Design review of the part built by this model. Coordinates are the model's own, in mm. A direction names the side the tool comes from. Coordinates: 2 decimals unless noted, no trailing zeros. Write each loop counter-clockwise with the first axis right and the second up, starting at its lowest first coordinate (ties: lowest second). Pieces come first, ordered by that corner, then holes. Notation, with made-up numbers: M -22.75,33 L 12.25,33 A26 cw 12.25,48 Z; hole C 35.25,-4 d7. An arc over 180 degrees is marked long. One line per question, with ' | ' between items.
from build123d import *

# Parameters (mm, degrees)
SKETCH1_W            = 30
SKETCH1_H            = 5
BOSS_EXTRUDE1_DEPTH  = 19.3
SKETCH2_W            = 40
SKETCH2_H            = 10
BOSS_EXTRUDE2_DEPTH  = 3.175
SKETCH3_W            = 4
SKETCH3_H            = 30
BOSS_EXTRUDE3_DEPTH  = 75
CUT_EXTRUDE1_REACH   = 84.48
SKETCH4_R            = 7.1
BOSS_EXTRUDE7_DEPTH  = 5
BOSS_EXTRUDE8_DEPTH  = 5
CHAMFER1_SIZE        = 5
BOSS_EXTRUDE9_DEPTH  = 75
BOSS_EXTRUDE10_DEPTH = 5
CHAMFER2_SIZE        = 5
CHAMFER3_SIZE        = 10
BOSS_EXTRUDE15_DEPTH = 3.175
CUT_EXTRUDE2_DEPTH   = 81.759021382
FILLET6_R            = 1
FILLET7_R            = 1
CHAMFER6_SIZE        = 2.5


with BuildPart() as part:
    # Sketch1 → Boss-Extrude1 (new body)
    with BuildSketch(Plane(origin=(0, 0, 0), x_dir=(0, 0, -1), z_dir=(1, 0, 0))):
        Rectangle(SKETCH1_W, SKETCH1_H)
    extrude(amount=BOSS_EXTRUDE1_DEPTH)

    # Sketch2 → Boss-Extrude2 (add)
    with BuildSketch(Plane.ZY):
        with Locations((0.597390222, 2.5)):
            Rectangle(SKETCH2_W, SKETCH2_H)
    extrude(amount=-BOSS_EXTRUDE2_DEPTH)

    # Sketch3 → Boss-Extrude3 (add)
    with BuildSketch(Plane.XZ.offset(2.5)):
        with Locations((17.3, 0)):
            Rectangle(SKETCH3_W, SKETCH3_H)
    extrude(amount=BOSS_EXTRUDE3_DEPTH)

    # Sketch4 → Cut-Extrude1 (cut, up to next)
    with BuildSketch(Plane(origin=(19.3, 0, 0), x_dir=(0, 0, -1), z_dir=(1, 0, 0)), mode=Mode.PRIVATE) as cut_extrude1_sk1:
        with Locations((2.035e-06, -17.9)):
            Circle(SKETCH4_R)
    cut_extrude1_tool1 = extrude(cut_extrude1_sk1.sketch, amount=-CUT_EXTRUDE1_REACH, mode=Mode.PRIVATE) & part.part
    # Sketch4 → Cut-Extrude1 (cut, up to next)
    with BuildSketch(Plane(origin=(19.3, 0, 0), x_dir=(0, 0, -1), z_dir=(1, 0, 0)), mode=Mode.PRIVATE) as cut_extrude1_sk2:
        with Locations((-1.3e-07, -65.9)):
            Circle(SKETCH4_R)
    cut_extrude1_tool2 = extrude(cut_extrude1_sk2.sketch, amount=-CUT_EXTRUDE1_REACH, mode=Mode.PRIVATE) & part.part
    add(cut_extrude1_tool1.solids().sort_by_distance((19.3, -17.9, -2e-06))[0], mode=Mode.SUBTRACT)
    add(cut_extrude1_tool2.solids().sort_by_distance((19.3, -65.9, 0))[0], mode=Mode.SUBTRACT)

    # Sketch10 → Boss-Extrude7 (add)
    with BuildSketch(Plane(origin=(0, 2.5, 0), x_dir=(1, 0, 0), z_dir=(0, 1, 0))):
        Polygon((3.175, 19.402609778), (0, 19.402609778), (0, 22.902609778), (19.3, 15), (3.175, 15), align=None)
    boss_extrude7 = extrude(amount=-BOSS_EXTRUDE7_DEPTH)

    # Sketch11 → Boss-Extrude8 (add)
    with BuildSketch(Plane(origin=(0, 2.5, 0), x_dir=(1, 0, 0), z_dir=(0, 1, 0))):
        Polygon((0, 19.402609778), (0, 22.902609778), (3.175, 21.60256905), (3.175, 19.402609778), align=None)
    boss_extrude8 = extrude(amount=BOSS_EXTRUDE8_DEPTH)

    # Mirror2: Boss-Extrude7, Boss-Extrude8 across plane
    add(boss_extrude7.mirror(Plane(origin=(0, 0, 0), x_dir=(1, 0, 0), z_dir=(0, 0, -1))))
    add(boss_extrude8.mirror(Plane(origin=(0, 0, 0), x_dir=(1, 0, 0), z_dir=(0, 0, -1))))

    # Chamfer1
    chamfer1_edges = [part.edges().sort_by_distance(p)[0] for p in [
        (3.175, 2.5, 0),
    ]]
    chamfer(chamfer1_edges, length=CHAMFER1_SIZE - 0.0001)  # a hair under: the kernel refuses the full size

    # Sketch12 → Boss-Extrude9 (add)
    with BuildSketch(Plane.XZ.offset(2.5)):
        Polygon((0, -22.902609778), (19.3, -15), (15.3, -15), (0, -21.264763192), align=None)
        Polygon((0, 22.902609778), (19.3, 15), (15.3, 15), (0, 21.264763192), align=None)
    extrude(amount=BOSS_EXTRUDE9_DEPTH)

    # Sketch13 → Boss-Extrude10 (add)
    with BuildSketch(Plane(origin=(0, 2.5, 0), x_dir=(1, 0, 0), z_dir=(0, 1, 0))):
        Polygon((3.175, 21.60256905), (3.175, -21.60256905), (19.3, -15), (19.3, 15), align=None)
    extrude(amount=BOSS_EXTRUDE10_DEPTH)

    # Chamfer2
    chamfer2_edges = [part.edges().sort_by_distance(p)[0] for p in [
        (7.65, -2.5, -18.132381596),
        (7.65, -2.5, 18.132381596),
        (15.3, -2.5, 0),
    ]]
    chamfer(chamfer2_edges, length=CHAMFER2_SIZE)

    # Chamfer3
    chamfer3_edges = [part.edges().sort_by_distance(p)[0] for p in [
        (9.65, 7.5, 18.951304889),
        (19.3, 7.5, 0),
        (9.65, 7.5, -18.951304889),
    ]]
    chamfer(chamfer3_edges, length=CHAMFER3_SIZE)

    # Sketch14 → Boss-Extrude15 (add)
    with BuildSketch(Plane.ZY):
        Polygon((-22.902609778, -2.5), (-22.902609778, 7.718772797), (-15.034642071, 15), (15.034642071, 15), (22.902609778, 7.718772797), (22.902609778, -2.5), align=None)
    extrude(amount=-BOSS_EXTRUDE15_DEPTH)

    # Sketch15 → Cut-Extrude2 (cut, through all)
    with BuildSketch(Plane.XZ.offset(2.5)):
        Polygon((3.175, 22.902609778), (0, 22.902609778), (3.175, 21.60256905), align=None)
        Polygon((3.175, -22.902609778), (3.175, -21.60256905), (0, -22.902609778), align=None)
    extrude(amount=-CUT_EXTRUDE2_DEPTH, mode=Mode.SUBTRACT)

    # Fillet6
    fillet6_edges = [part.edges().sort_by_distance(p)[0] for p in [
        (9.3, 7.5, 0),
        (6.2375, 7.5, -9.542766367),
        (6.2375, 7.5, 9.542766367),
    ]]
    fillet(fillet6_edges, radius=FILLET6_R)

    # Fillet7
    fillet7_edges = [part.edges().sort_by_distance(p)[0] for p in [
        (11.2375, -2.5, 18.301284525),
        (19.3, -2.5, 0),
        (11.2375, -2.5, -18.301284525),
    ]]
    fillet(fillet7_edges, radius=FILLET7_R)

    # Chamfer6
    chamfer6_edges = [part.edges().sort_by_distance(p)[0] for p in [
        (9.65, -77.5, -18.951304889),
        (19.3, -77.5, 0),
        (9.65, -77.5, 18.951304889),
    ]]
    chamfer(chamfer6_edges, length=CHAMFER6_SIZE)


solid = part.part
1. Take a section at B-B (z = 0). Write out the cut boundary in (x, y) (3 decimals), then the cut area to 3 significant figures.
Answer sheet:
outline: M 0,-2.5 L 10.3,-2.5 L 15.3,-7.5 L 15.3,-10.8 L 19.3,-10.8 L 19.3,-2.914 A1 ccw 19.007,-2.207 L 9.593,7.207 A1 ccw 8.886,7.5 L 3.175,7.5 L 3.175,15 L 0,15 Z; M 15.3,-77.5 L 16.8,-77.5 L 19.3,-75 L 19.3,-73 L 15.3,-73 Z; M 15.3,-58.8 L 19.3,-58.8 L 19.3,-25 L 15.3,-25 Z | area: 363 mm^2
2. Take a section at C-C (y = -38.5). Write out the cut boundary in (x, z).
Answer sheet:
outline: M 0,-22.9 L 19.3,-15 L 19.3,15 L 0,22.9 L 0,21.26 L 15.3,15 L 15.3,-15 L 0,-21.26 Z
3. Take a section at D-D (x = 18). Count the separate pieces of the cut face and the enclosed holes in it, then the cut area to 3 significant figures.
Answer sheet:
separate pieces: 1 | enclosed holes: 2 | area: 2,010 mm^2
4. Draft analysis for pull direction Z (two halves, no side actions). For faces 1 (the face through (9.25, -75.71, -18.35)), 2 (the face through (7.757, -41.525, -18.089)), 3 (the face through (3.175, 8, 0)), state which applies: pulls with the +Z half, pulls with the -Z half, needs draft (parallel to the pull), parting line crosses it, or undercut.
Answer sheet:
face 1: pulls with the -Z half | face 2: undercut | face 3: needs draft
5. Insertion check: pin 1 Ø8 at (x, z) = (3.5, 14) entering from -Y; pin 2 Ø8 at (x, z) = (7, 3.5) entering from -Y; pin 3 Ø1 at (x, z) = (6, 1) entering from +Y. Each pin has a flat end and moves straight along its axis. Give the tip position at first contact, or say it passes through.
Answer sheet:
pin 1: y = -6.1 | pin 2: y = -3.2 | pin 3: y = 7.5
6. Take a section at A-A (y = -17.9). Write out the cut boundary in (x, z), then the cut area to 3 significant figures.
Answer sheet:
outline: M 0,-22.9 L 19.3,-15 L 19.3,-7.1 L 15.3,-7.1 L 15.3,-15 L 0,-21.26 Z; M 0,21.26 L 15.3,15 L 15.3,7.1 L 19.3,7.1 L 19.3,15 L 0,22.9 Z | area: 120 mm^2
7. Tool access review of faces 4 (the face through (6.797, -4.965, 15.743)), 5 (the face through (0, 0, 2)), 6 (the face through (6, 7.5, 0)): name each direction out of +Z, -Z, +X, -X, +Y, -Y from which nothing blocks a thin tool from reaching the whole face with its end or side.
Answer sheet:
face 4: -X, -Y | face 5: +Z, -Z, -X, +Y, -Y | face 6: +Z, -Z, +X, +Y
8. To check wall thickness, follow line 1 along Y through (x, z) = (17.4, 0); line 2 along Y through (x, z) = (2.5, 6); line 3 along Z through (x, y) = (8.5, -6). State the ranges of each line that lie inside material, in increasing order. Write a range as [from, to].
Answer sheet:
line 1: [-76.9, -73], [-58.8, -25], [-10.8, -0.6] | line 2: [-2.5, 15] | line 3: [-19.42, -16.16], [16.16, 19.42]
